```python
from build123d import *

# Parameters (mm, degrees)
SKETCH1_R           = 1.25
BOSS_EXTRUDE1_DEPTH = 10
SKETCH2_W           = 3
SKETCH2_H           = 8.5
CUT_EXTRUDE1_DEPTH  = 6
SKETCH3_W           = 5
SKETCH3_H           = 26
SKETCH3_R           = 1.15
BOSS_EXTRUDE2_DEPTH = 3
CHAMFER1_SIZE       = 2
CHAMFER1_SIZE2      = 4
CHAMFER2_SIZE       = 4
CHAMFER2_SIZE2      = 2


with BuildPart() as part:
    # Sketch1 → Boss-Extrude1 (new body)
    with BuildSketch(Plane.XY):
        with BuildLine():
            Line((2.5, 15), (2.5, 0))
            Line((2.5, 0), (-2.5, 0))
            Line((-2.5, 0), (-2.5, 15))
            ThreePointArc((-2.5, 15), (0, 15.877501001), (2.5, 15))
        make_face()
        with Locations((0, 11.877501001)):
            Circle(SKETCH1_R, mode=Mode.SUBTRACT)
    extrude(amount=-BOSS_EXTRUDE1_DEPTH)

    # Sketch2 → Cut-Extrude1 (cut, through all)
    with BuildSketch(Plane.ZY.offset(2.5)):
        with Locations((-5, 11.627501001)):
            Rectangle(SKETCH2_W, SKETCH2_H)
    extrude(amount=-CUT_EXTRUDE1_DEPTH, mode=Mode.SUBTRACT)

    # Sketch3 → Boss-Extrude2 (add)
    with BuildSketch(Plane.XZ):
        with Locations((0, -5)):
            Rectangle(SKETCH3_W, SKETCH3_H)
        with Locations((0, 5)):
            Circle(SKETCH3_R, mode=Mode.SUBTRACT)
        with Locations((0, -15)):
            Circle(SKETCH3_R, mode=Mode.SUBTRACT)
    extrude(amount=-BOSS_EXTRUDE2_DEPTH)

    # Chamfer1
    chamfer1_edges = [part.edges().sort_by_distance(p)[0] for p in [
        (0, 3, -10),
    ]]
    chamfer1_side = [part.faces().sort_by_distance(p)[0] for p in [
        (-2.405660189, 3, -14),
    ]]
    chamfer(chamfer1_edges, length=CHAMFER1_SIZE, length2=CHAMFER1_SIZE2, reference=chamfer1_side[0])

    # Chamfer2
    chamfer2_edges = [part.edges().sort_by_distance(p)[0] for p in [
        (0, 3, 0),
    ]]
    chamfer2_side = [part.faces().sort_by_distance(p)[0] for p in [
        (0, 9.084568634, 0),
    ]]
    chamfer(chamfer2_edges, length=CHAMFER2_SIZE, length2=CHAMFER2_SIZE2, reference=chamfer2_side[0])


solid = part.part
```
Geometry: final body of the model. Coordinates: model frame, mm. A direction names the side the tool comes from. Give positions to 0.01 mm unless a question says otherwise; leave off trailing zeros. Order: outer loops, then holes, each group sorted by start corner. A loop starts at its lowest first (then second) coordinate and runs counter-clockwise, first axis right, second up. Notation, with made-up numbers: (79, 83.25) -> (126, 83.25) arc R18 ccw to (126, 116.25) -> close; hole circle Ø6 at (11.5, 84.5). An arc over 180 degrees is marked (long way). Write each question's results on one line, items separated by ' | '. Start each with the question number.
1) Draft query along X for faces 5 (the flat face through (0.6, 10.5, 0)), 6 (the cylindrical face through (-0.163, 13.117, -8.226)), 7 (the flat face through (2.5, 4, -5)). Return one class per face: pulls with the +X half, pulls with the -X half, needs draft (parallel to the pull), parting line crosses it, or undercut.
2) First-contact query: pin 1 (2 mm diameter, centred on x = 0, z = 5, fed in from +Y); pin 2 (2.5 mm diameter, centred on x = 0.5, y = 13, fed in from -Z); pin 3 (1 mm diameter, centred on x = -1.5, y = 6, fed in from +Z); pin 4 (2.5 mm diameter, centred on x = -0.5, y = 12.5, fed in from +Z). Flat tips, straight axial feed; report the tip coordinate or a pass-through.
3) Section B-B (x = 0). Count the separate pieces of the cut face and the enclosed holes in it, then the cut area to 3 significant figures.
4) Section A-A (z = 5). Return loops of the section in (x, y), then the cut area to 3 significant figures.
5) Line query: line 1 (Z direction, x = 1.3, y = 8.75); line 2 (Z direction, x = -1.05, y = 2.25); line 3 (Y direction, x = -1.1, z = -13). Output: solid intervals per line, ascending. Write a range as from..to.
6) Set-up query: faces 1 (the flat face through (-0.6, 10.6, -3.5)), 2 (the flat face through (0.6, 10.5, -10)), 3 (the flat face through (1, 3, 4)), 4 (the cylindrical face through (-0.15, 1.48, 6.14)). Return all of +Z, -Z, +X, -X, +Y, -Y with unobstructed straight access to the full face (end or side cutting, diameter ignored); none if empty.
7) Section C-C (y = 15.25). Return loops of the section in (x, z), then the cut area to 3 significant figures.
8) Section D-D (z = -16.5). Return loops of the section in (x, y), then the cut area to 3 significant figures.
Calculated:
1) face 5: needs draft | face 6: undercut | face 7: pulls with the +X half
2) pin 1: through | pin 2: z = -10 | pin 3: z = 0.75 | pin 4: z = 0
3) separate pieces: 5 | enclosed holes: 0 | area: 158 mm2
4) outline: (-2.5, 0) -> (-1.15, 0) -> (-1.15, 3) -> (-2.5, 3) -> close; (1.15, 0) -> (2.5, 0) -> (2.5, 3) -> (1.15, 3) -> close | area: 8.10 mm2
5) line 1: -10..-6.5, -3.5..0 | line 2: -18..-15.47, -14.53..4.53, 5.47..8 | line 3: 0..3
6) face 1: +X, -X, +Y | face 2: -Z, +X, -X, +Y | face 3: +Z, +X, -X, +Y | face 4: +Y, -Y
7) outline: (-2.15, -10) -> (2.15, -10) -> (2.15, -6.5) -> (-2.15, -6.5) -> close; (-2.15, -3.5) -> (2.15, -3.5) -> (2.15, 0) -> (-2.15, 0) -> close | area: 30.1 mm2
8) outline: (-2.5, 0) -> (2.5, 0) -> (2.5, 3) -> (-2.5, 3) -> close | area: 15.0 mm2
